from build123d import *

# Parameters (mm, degrees)
SKETCH_W     = 30
SKETCH_H     = 93
PAD_DEPTH    = 3
SKETCH001_W  = 7
SKETCH001_H  = 7
SKETCH001_R  = 1.5
PAD001_DEPTH = 7
SKETCH002_R  = 2.2
HOLE_DEPTH   = 25
CHAMFER_SIZE = 11


with BuildPart() as part:
    # Sketch → Pad (new body)
    with BuildSketch(Plane.XY):
        with Locations((0, 46.5)):
            Rectangle(SKETCH_W, SKETCH_H)
    extrude(amount=PAD_DEPTH)

    # Sketch001 (on Face6 of Pad) → Pad001 (join)
    with BuildSketch(Plane.XY.offset(3)):
        with Locations((0, 3.5)):
            Rectangle(SKETCH001_W, SKETCH001_H)
        with Locations((0, 3.5)):
            Circle(SKETCH001_R, mode=Mode.SUBTRACT)
        with Locations((-11.5, 89.5)):
            Rectangle(SKETCH001_W, SKETCH001_H)
        with Locations((-11.5, 89.5)):
            Circle(SKETCH001_R, mode=Mode.SUBTRACT)
        with Locations((11.5, 89.5)):
            Rectangle(SKETCH001_W, SKETCH001_H)
        with Locations((11.5, 89.5)):
            Circle(SKETCH001_R, mode=Mode.SUBTRACT)
    extrude(amount=PAD001_DEPTH)

    # Sketch002 (on Face6 of Pad001) → Hole (cut)
    with BuildSketch(Plane.XY.offset(3)):
        with Locations((0, 61.5)):
            Circle(SKETCH002_R)
        with Locations((0, 31.5)):
            Circle(SKETCH002_R)
    extrude(amount=-HOLE_DEPTH, mode=Mode.SUBTRACT)

    # Chamfer
    chamfer_edges = [part.edges().sort_by_distance(p)[0] for p in [
        (15, 0, 1.5),
        (-15, 0, 1.5),
    ]]
    chamfer(chamfer_edges, length=CHAMFER_SIZE)


solid = part.part
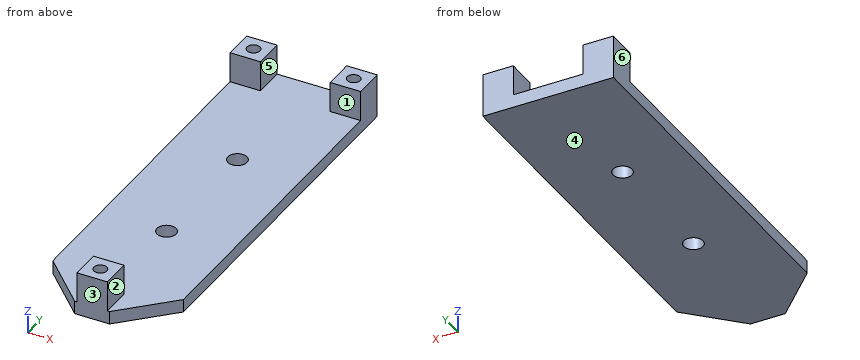
Design review of the part built by this model. Coordinates are the model's own, in mm. Face numbers are marked on the shaded views. A direction names the side the tool comes from. Round coordinates to 2 decimals unless told otherwise and drop trailing zeros. Write each loop counter-clockwise with the first axis right and the second up, starting at its lowest first coordinate (ties: lowest second). Pieces come first, ordered by that corner, then holes.
Item 1: For the marked faces 1, 2 and 3, list the 3-axis set-ups (+Z, -Z, +X, -X, +Y, -Y) from which the entire face can be reached by the end or side of a thin tool; tool diameter is ignored.
Item 2: Consider section A-A on y = 31.5. Give the boundary of the cut face in (x, z), and give its area (3 significant figures).
Item 3: For pin 1 Ø15 at (x, y) = (-1, 57) entering from +Z; pin 2 Ø3.5 at (x, z) = (-11.5, 7) entering from -Y; pin 3 Ø1.5 at (x, z) = (-6, 1) entering from -Y, all flat-tipped, find the tip position at first contact; note any pin that passes through.
Item 4: Wall thickness on L1, parallel to X at y = 89.5, z = 7.25; L2, parallel to Y at x = 0, z = 5; L3, parallel to Y at x = -11.5, z = 8.5: over which ranges is each line inside the solid? List them lowest first.
Item 5: Consider section C-C on z = 6.5. Give the boundary of the cut face in (x, y).
Item 6: Draft analysis for pull direction X (two halves, no side actions). For the marked faces 4, 5 and 6, state which applies: released by +X, released by -X, zero draft, split by the parting line, or undercut.
Item 7: Consider section D-D on y = 89.5. Give the boundary of the cut face in (x, z), and give its area (3 significant figures).
Item 8: Consider section B-B on z = 1. Give the boundary of the cut face in (x, y), and give its area (3 significant figures).
Check values:
1. face 1: +Z, +X, -X, -Y
1. face 2: +Z, +X, +Y, -Y
1. face 3: +Z, -Z, +X, -X, -Y
2. outline: (-15, 0) - (-2.2, 0) - (-2.2, 3) - (-15, 3) - close; (2.2, 0) - (15, 0) - (15, 3) - (2.2, 3) - close
2. area: 76.8 mm2
3. pin 1: stops at z = 3
3. pin 2: stops at y = 86
3. pin 3: stops at y = 1.25
4. L1: x = -15 to -13, -10 to -8, 8 to 10, 13 to 15
4. L2: y = 0 to 2, 5 to 7
4. L3: y = 86 to 88, 91 to 93
5. outline: (-15, 86) - (-8, 86) - (-8, 93) - (-15, 93) - close; (-3.5, 0) - (3.5, 0) - (3.5, 7) - (-3.5, 7) - close; (8, 86) - (15, 86) - (15, 93) - (8, 93) - close; hole circle Ø3 at (-11.5, 89.5); hole circle Ø3 at (0, 3.5); hole circle Ø3 at (11.5, 89.5)
6. face 4: zero draft
6. face 5: undercut
6. face 6: released by -X
7. outline: (-15, 0) - (15, 0) - (15, 10) - (13, 10) - (13, 3) - (10, 3) - (10, 10) - (8, 10) - (8, 3) - (-8, 3) - (-8, 10) - (-10, 10) - (-10, 3) - (-13, 3) - (-13, 10) - (-15, 10) - close
7. area: 146 mm2
8. outline: (-15, 11) - (-4, 0) - (4, 0) - (15, 11) - (15, 93) - (-15, 93) - close; hole circle Ø4.4 at (0, 31.5); hole circle Ø4.4 at (0, 61.5)
8. area: 2,640 mm2
